Can you work these out from the drawing? Everything is in mm from the part's minimum corner. A direction names the side the tool comes from. Coordinates: 2 decimals unless noted, no trailing zeros. Order: outer loops, then holes, each group sorted by start corner. A loop starts at its lowest first (then second) coordinate and runs counter-clockwise, first axis right, second up. Notation, with made-up numbers: (3, -6) -> (16, -6) arc R19 cw to (16, 16) -> close; hole circle Ø5 at (-39, 6.25). An arc over 180 degrees is marked (long way). Answer in a Markdown table with one row per item.
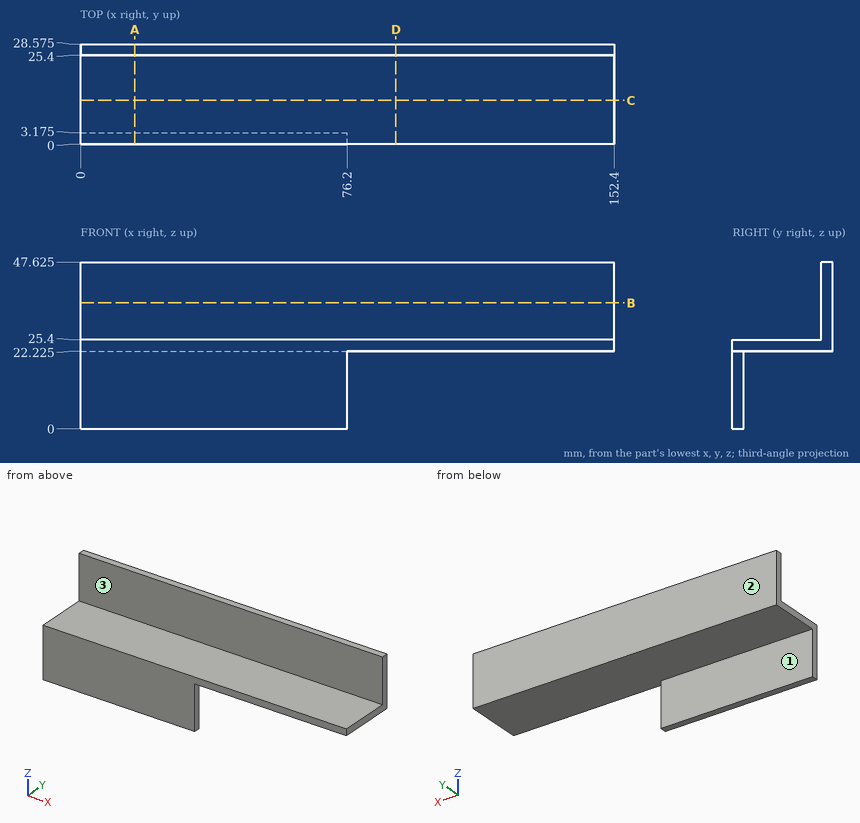
(1) Will these pins go through, and if not, where does the flat tip stop? pin 1 Ø4 at (x, y) = (87.5, 6.5) entering from +Z; pin 2 Ø3 at (x, z) = (125.5, 27.5) entering from -Y; pin 3 Ø2.5 at (y, z) = (1.5, 7) entering from +X.
Response values:
| item | result |
|---|---|
| pin 1 | z = 25.4 |
| pin 2 | y = 25.4 |
| pin 3 | x = 76.2 |
(2) I need wall thicknesses on line 1 (Z direction, x = 61.5, y = 12) (3 decimals); line 2 (Z direction, x = 106, y = 26) (3 decimals); line 3 (Y direction, x = 72.5, z = 19.5) (3 decimals). Which ranges of each line are inside material? Lowest first, please. Write a range as [from, to].
Response values:
| item | result |
|---|---|
| line 1 | [22.225, 25.4] |
| line 2 | [22.225, 47.625] |
| line 3 | [0, 3.175] |
(3) On a 3-axis mill with a long thin cutter (end or side, diameter ignored), from which of +Z, -Z, +X, -X, +Y, -Y can I reach the whole of each face in a straight line? I mean the marked faces 1, 2 and 3. Say none if no direction works.
Response values:
| item | result |
|---|---|
| face 1 | -Z, +X, -X, +Y |
| face 2 | +Z, -Z, +X, -X, +Y |
| face 3 | +Z, +X, -X, -Y |
(4) Suppose I cut it at B-B (z = 36). Please give me the cut outline in (x, y) (3 decimals), and give its area (3 significant figures).
Response values:
| item | result |
|---|---|
| outline | (0, 25.4) -> (152.4, 25.4) -> (152.4, 28.575) -> (0, 28.575) -> close |
| area | 484 mm2 |
(5) Suppose I cut it at C-C (y = 12.5). Please give me the cut outline in (x, z) (3 decimals), and give its area (3 significant figures).
Response values:
| item | result |
|---|---|
| outline | (0, 22.225) -> (152.4, 22.225) -> (152.4, 25.4) -> (0, 25.4) -> close |
| area | 484 mm2 |
(6) Suppose I cut it at A-A (x = 15.5). Please give me the cut outline in (y, z) (3 decimals).
Response values:
| item | result |
|---|---|
| outline | (0, 0) -> (3.175, 0) -> (3.175, 22.225) -> (28.575, 22.225) -> (28.575, 47.625) -> (25.4, 47.625) -> (25.4, 25.4) -> (0, 25.4) -> close |
(7) Suppose I cut it at D-D (x = 90). Please give me the cut outline in (y, z) (3 decimals), and give its area (3 significant figures).
Response values:
| item | result |
|---|---|
| outline | (0, 22.225) -> (28.575, 22.225) -> (28.575, 47.625) -> (25.4, 47.625) -> (25.4, 25.4) -> (0, 25.4) -> close |
| area | 161 mm2 |
